Here's how the part is built. I have some questions about the finished solid (model axes, mm). A direction names the side the tool comes from. Round coordinates to 2 decimals unless told otherwise and drop trailing zeros. Write each loop counter-clockwise with the first axis right and the second up, starting at its lowest first coordinate (ties: lowest second). Pieces come first, ordered by that corner, then holes. Notation, with made-up numbers: (87.25, -34.75) - (93.25, -34.75) arc R34 cw to (93.25, -1.75) - close; hole circle Ø2 at (6.25, 22.25). An arc over 180 degrees is marked (long way). Write item = value, one per line. Start each with the question number.
Item 1: For P1, Ø1.5, axis at x = 3, z = 8.5, coming from the -Y side; P2, Ø3, axis at y = 7, z = 7, coming from the -X side; P3, Ø1.5, axis at x = 8, y = -5.5, coming from the -Z side, each with a flat end and sliding along its axis, tell me the tip position at first contact or that it passes through.
Item 2: If we section it at A-A (z = 5.25): Please give me the cut outline in (x, y), and give its area (3 significant figures).
Item 3: Thinking about a two-plate mould opening in Y: for faces 1 (the face through (2, 14, 13)), 2 (the face through (7.1, 0, 1)), 3 (the face through (11.159, -9.036, 8.437)), which applies, pulls with the +Y half, pulls with the -Y half, needs draft (parallel to the pull), parting line crosses it, or undercut?
Item 4: If I drill on line 1 along Y through (x, z) = (0, 5.5); line 2 along Y through (x, z) = (-2, 7.75); line 3 along X through (y, z) = (1.5, 8.5), over which ranges is the centre line in solid material (lowest first)? Write a range as [from, to].
Item 5: Which directions (+Z, -Z, +X, -X, +Y, -Y) give clear straight access to the entire face, cutting with the end or side of a thin tool? Please do faces 4 (the face through (-0.1, -13.7, 8.4)), 5 (the face through (5.14, -13.39, 8.44)), 6 (the face through (-5.146, -13.405, 8.437)), 7 (the face through (2, -6, 2.5)).
```python
from build123d import *

# Parameters (mm, degrees)
CUT_EXTRUDE4_DEPTH = 2.5
CUT_REVOLVE1_START = 4
CUT_REVOLVE1_DEPTH = 9
CIRPATTERN1_COUNT  = 5


# Read off the part's stored shape, not the designer's step: Cut-Revolve1
with BuildPart() as part:
    # Sketch1 → Revolve1 (revolve)
    with BuildSketch(Plane(origin=(0, 0, 0), x_dir=(1, 0, 0), z_dir=(0, 1, 0)), mode=Mode.PRIVATE) as revolve1_sk:
        with BuildLine():
            Line((6.15, -10.15), (6.15, 0))
            ThreePointArc((6.15, 0), (10.822325438, -0.770389957), (15, -3))
            Line((15, -3), (15, -13))
            Line((15, -13), (13.7, -13))
            Line((13.7, -13), (13.7, -4))
            Line((13.7, -4), (11.4, -4))
            Line((11.4, -4), (11.4, -13))
            Line((11.4, -13), (8, -13))
            Line((8, -13), (8, -12))
            Line((8, -12), (6.15, -10.15))
        make_face()
    revolve(revolve1_sk.sketch.rotate(Axis((0, 0, 0), (0, 0, 1)), 180), axis=Axis((0, 0, 0), (0, 0, 1)))

    # Sketch7 → Cut-Extrude4 (cut)
    with BuildSketch(Plane.XY):
        Polygon((0, -8.198373822), (7.1, -4.099186911), (7.1, 4.099186911), (0, 8.198373822), (-7.1, 4.099186911), (-7.1, -4.099186911), align=None)
    extrude(amount=CUT_EXTRUDE4_DEPTH, mode=Mode.SUBTRACT)

    # Cut-Revolve1 outline → Cut-Revolve1 (cut)
    with BuildSketch(Plane.XY.offset(CUT_REVOLVE1_START)):
        with BuildLine():
            Line((11.657189422, -9.439805866), (10.646899672, -8.621689357))
            ThreePointArc((10.646899672, -8.621689357), (8.052657957, -11.083532823), (4.909640909, -12.790051843))
            Line((4.909640909, -12.790051843), (5.375519243, -14.003706397))
            ThreePointArc((5.375519243, -14.003706397), (8.816778784, -12.135254916), (11.657189422, -9.439805866))
        make_face()
    cut_revolve1 = extrude(amount=CUT_REVOLVE1_DEPTH, mode=Mode.SUBTRACT)

    # CirPattern1: Cut-Revolve1 ×5 about axis, 3 skipped
    cirpattern1_axis = Axis((0, 0, -1.227748989), (0, 0, 1))
    add([cut_revolve1.rotate(cirpattern1_axis, i * 360 / CIRPATTERN1_COUNT) for i in range(1, CIRPATTERN1_COUNT) if i not in (1, 2, 3)], mode=Mode.SUBTRACT)


solid = part.part
```
Reply:
q1.P1 = -14.83
q1.P2 = -13.96
q1.P3 = 0.27
q2.outline = (-11.66, -9.44) - (-10.65, -8.62) arc R13.7 cw (long way) to (10.65, -8.62) - (11.66, -9.44) arc R15 ccw (long way) to start; circle Ø22.8 at (0, 0); (-5.38, -14) arc R15 ccw to (5.38, -14) - (4.91, -12.79) arc R13.7 cw to (-4.91, -12.79) - close; hole circle Ø12.3 at (0, 0)
q2.area = 387 mm2
q3.face_1 = needs draft
q3.face_2 = undercut
q3.face_3 = pulls with the -Y half
q4.line_1 = [-15, -13.7], [-11.4, -6.15], [6.15, 11.4], [13.7, 15]
q4.line_2 = [-14.87, -13.55], [-11.22, -5.82], [5.82, 11.22], [13.55, 14.87]
q4.line_3 = [-14.92, -13.62], [-11.3, -5.96], [5.96, 11.3], [13.62, 14.92]
q5.face_4 = +Z
q5.face_5 = +Z, +X
q5.face_6 = +Z, -X
q5.face_7 = -Z
